Answer from the drawing. Dimensions are ordinates in mm from the lowest x, y and z of the part. A direction names the side the tool comes from. Coordinates: 2 decimals unless noted, no trailing zeros. Order: outer loops, then holes, each group sorted by start corner. A loop starts at its lowest first (then second) coordinate and runs counter-clockwise, first axis right, second up. Notation, with made-up numbers: M 51.25,4 L 56.25,4 A26 ccw 56.25,35 Z; hole C 70.25,51 d1. An arc over 180 degrees is marked long. One line per question, with ' | ' between items. Start each with the question number.
1) Find section D-D, the plane z = 24.75. Write down the section's boundary in (x, y), plus the area to 3 significant figures.
2) Given P1, Ø1, axis at x = 9.5, y = 10.5, coming from the +Z side; P2, Ø4, axis at y = 16, z = 24.5, coming from the -X side, each flat-ended and moving along its own axis, determine where each tip first touches the part or whether it passes through.
3) Find section A-A, the plane x = 6.25. Write down the section's boundary in (y, z).
4) Consider probe 1 along Z at (x, y) = (4, 9.25); probe 2 along X at (y, z) = (16.5, 23.75); probe 3 along X at (y, z) = (16.5, 27.5). Determine where each line is inside the solid, lowest interval first.
5) A tool of negligible diameter and unlimited length cuts with its end or side. For the marked faces 1 and 2, from which of +Z, -Z, +X, -X, +Y, -Y can it reach the whole face along a straight path? Write none if from no direction.
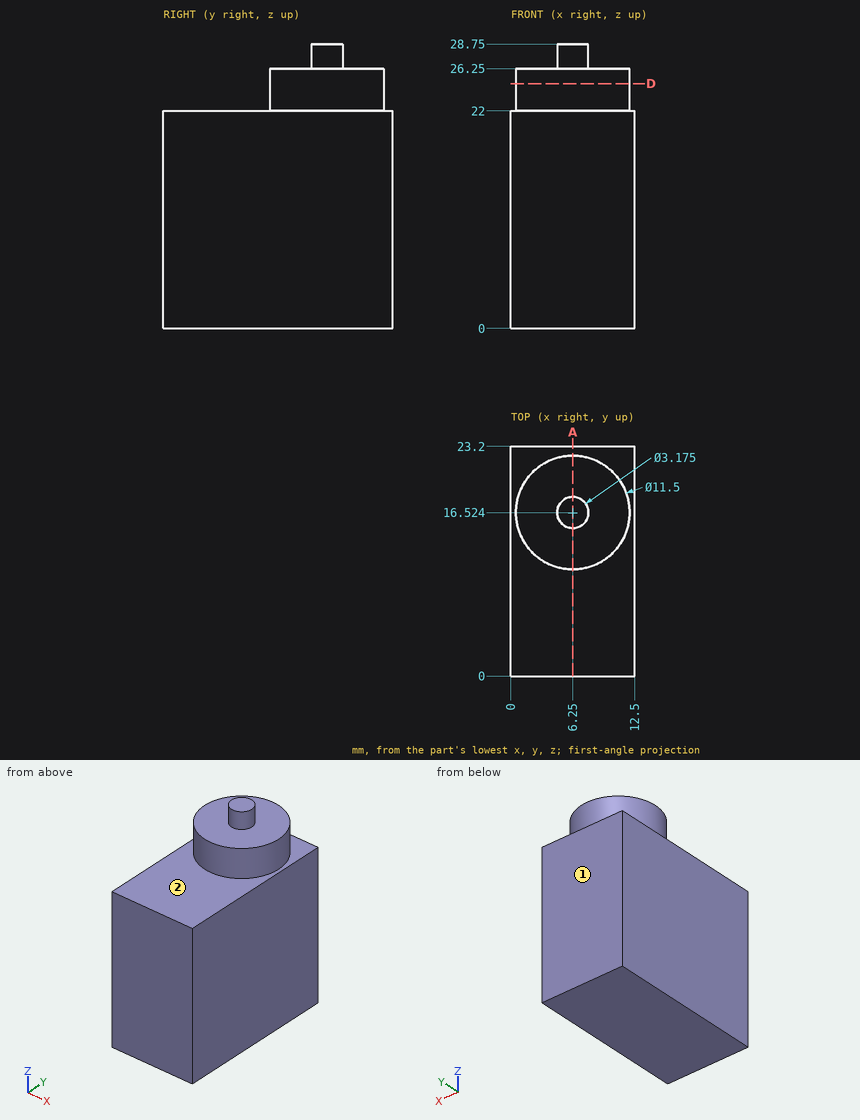
Report:
1) outline: C 6.25,16.52 d11.5 | area: 104 mm^2
2) P1: stops at z = 22 | P2: stops at x = 0.5
3) outline: M 0,0 L 23.2,0 L 23.2,22 L 22.27,22 L 22.27,26.25 L 18.11,26.25 L 18.11,28.75 L 14.94,28.75 L 14.94,26.25 L 10.77,26.25 L 10.77,22 L 0,22 Z
4) probe 1: z = 0 to 22 | probe 2: x = 0.5 to 12 | probe 3: x = 4.66 to 7.84
5) face 1: +Z, -Z, +X, -X, +Y | face 2: +Z
